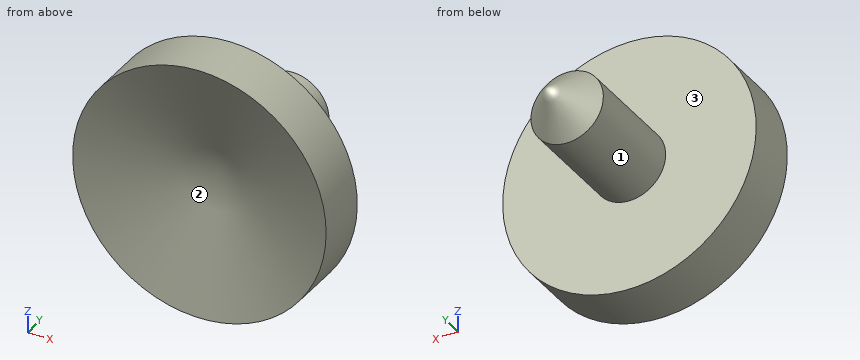
from build123d import *

# Parameters (mm, degrees)
BOSS_EXTRUDE1_START = 0.5
SKETCH1_R           = 3.5
BOSS_EXTRUDE1_DEPTH = 1.5
SKETCH5_R           = 1
BOSS_EXTRUDE2_DEPTH = 4
CHAMFER1_SIZE       = 1


# Read off the part's stored shape, not the designer's step: Cut-Loft1
with BuildPart() as part:
    # Sketch1 → Boss-Extrude1 (new body)
    with BuildSketch(Plane(origin=(0, 0, 0), x_dir=(1, 0, 0), z_dir=(0, 1, 0)).offset(BOSS_EXTRUDE1_START)):
        with Locations(Location((0, 0, 0), (0, 0, 270))):
            Circle(SKETCH1_R)
    extrude(amount=-BOSS_EXTRUDE1_DEPTH)

    # Cut-Loft1 outline → Cut-Loft1 (revolve, cut)
    with BuildSketch(Plane.XY):
        Polygon((3.5, -1), (0, 0), (0, -1), align=None)
    revolve(axis=Axis((0, 0, 0), (0, 1, 0)), mode=Mode.SUBTRACT)

    # Sketch5 → Boss-Extrude2 (add)
    with BuildSketch(Plane(origin=(0, 0.5, 0), x_dir=(1, 0, 0), z_dir=(0, 1, 0))):
        with Locations(Location((0, 0, 0), (0, 0, 270))):
            Circle(SKETCH5_R)
    extrude(amount=BOSS_EXTRUDE2_DEPTH)

    # Chamfer1
    chamfer1_edges = [part.edges().sort_by_distance(p)[0] for p in [
        (0, 4.5, -1),
    ]]
    chamfer(chamfer1_edges, length=CHAMFER1_SIZE)


solid = part.part
Geometry: final body of the model. Coordinates: model frame, mm. Face numbers are marked on the shaded views. Give positions to 0.01 mm unless a question says otherwise; leave off trailing zeros. Write each loop counter-clockwise with the first axis right and the second up, starting at its lowest first coordinate (ties: lowest second). Pieces come first, ordered by that corner, then holes. Notation, with made-up numbers: (50.25, 13) - (63.25, 13) arc R12 ccw to (63.25, 23) - close; hole circle Ø4 at (81, 42.25). An arc over 180 degrees is marked (long way). Return JSON: item names as keys, results as strings. Group by question number.
1) Mould query, pull axis X, two halves, no side actions, for the marked faces 1, 2 and 3. Classes: released by +X, released by -X, zero draft, split by the parting line, or undercut.
2) Section B-B on y = 1.6. Return the cut outline in (x, z).
3) First-contact query: P1, Ø4, axis at x = -2, z = 0, coming from the -Y side; P2, Ø2, axis at x = 0, z = -1.5, coming from the +Y side. Flat tips, straight axial feed; report the tip coordinate or a pass-through.
4) Line query: line 1 (X direction, y = 0.7, z = 0); line 2 (X direction, y = 1.6, z = -0.5); line 3 (Y direction, x = 0.75, z = -2.75). Output: solid intervals per line, ascending.
5) Section A-A on y = 0.2. Return the cut outline in (x, z).
Filled in:
{
 "1": {"face 1": "split by the parting line", "face 2": "undercut", "face 3": "zero draft"},
 "2": {"outline": "circle Ø2 at (0, 0)"},
 "3": {"P1": "stops at y = -1", "P2": "stops at y = 4"},
 "4": {"line 1": "x = -1 to 1", "line 2": "x = -0.87 to 0.87", "line 3": "y = -0.81 to 0.5"},
 "5": {"outline": "circle Ø7 at (0, 0)"}
}
